from build123d import *

# Parameters (mm, degrees)
SKETCH1_R           = 2.921
SKETCH1_R_2         = 14.0335
SKETCH1_R_3         = 10.8585
SKETCH1_R_4         = 2.4892
SKETCH1_R_5         = 12.3825
BOSS_EXTRUDE1_DEPTH = 6.35
SKETCH2_W           = 6.35
SKETCH2_H           = 6.35
SKETCH2_H_2         = 16.217729686
SKETCH2_R           = 2.15265
CUT_EXTRUDE2_DEPTH  = 196.570791382
FILLET1_R           = 2.54


with BuildPart() as part:
    # Sketch1 → Boss-Extrude1 (new body)
    with BuildSketch(Plane(origin=(0, 0, 0), x_dir=(1, 0, 0), z_dir=(0, 1, 0))):
        with BuildLine():
            ThreePointArc((-168.788743889, 72.590962133), (-181.488743889, 59.890962122), (-168.788743866, 47.190962133))
            Line((-168.788743866, 47.190962133), (-145.58139547, 45.094655563))
            Line((-145.58139547, 45.094655563), (-93.510572414, -45.094655563))
            Line((-93.510572414, -45.094655563), (-105.98261767, -48.892439505))
            ThreePointArc((-105.98261767, -48.892439505), (-111.899875664, -63.177964006), (-99.63261767, -72.590962133))
            Line((-99.63261767, -72.590962133), (47.56445351, -72.590962133))
            Line((47.56445351, -72.590962133), (47.56445351, 72.590962133))
            Line((47.56445351, 72.590962133), (-168.788743889, 72.590962133))
        make_face()
        with Locations(Location((-168.788743889, 59.890962133, 0), (0, 0, 270))):
            Circle(SKETCH1_R, mode=Mode.SUBTRACT)
        with Locations(Location((20.56425351, -34.490962133, 0), (0, 0, 270))):
            Circle(SKETCH1_R_2, mode=Mode.SUBTRACT)
        with Locations(Location((-22.22178223, -28.671379192, 0), (0, 0, 270))):
            Circle(SKETCH1_R_3, mode=Mode.SUBTRACT)
        with Locations(Location((-62.44294649, -9.090962133, 0), (0, 0, 270))):
            Circle(SKETCH1_R_4, mode=Mode.SUBTRACT)
        with Locations(Location((-62.44294649, -34.490962133, 0), (0, 0, 270))):
            Circle(SKETCH1_R_5, mode=Mode.SUBTRACT)
        with Locations(Location((-62.44294649, -59.890962133, 0), (0, 0, 270))):
            Circle(SKETCH1_R_4, mode=Mode.SUBTRACT)
        with Locations(Location((-99.63261767, -59.890962133, 0), (0, 0, 270))):
            Circle(SKETCH1_R, mode=Mode.SUBTRACT)
    extrude(amount=BOSS_EXTRUDE1_DEPTH)

    # Sketch2 → Cut-Extrude2 (cut, through all)
    with BuildSketch(Plane(origin=(0, 6.35, 0), x_dir=(1, 0, 0), z_dir=(0, 1, 0))):
        Polygon((47.56445351, 66.240962133), (41.21445351, 66.240962133), (41.21445351, 50.023232447), (41.21445351, 43.673232447), (41.21445351, -29.703590933), (47.56445351, -39.813704084), align=None)
        with Locations((44.38945351, 69.415962133)):
            Rectangle(SKETCH2_W, SKETCH2_H)
        with Locations((38.03945351, 58.13209729)):
            Rectangle(SKETCH2_W, SKETCH2_H_2)
        with Locations((38.03945351, 69.415962133)):
            Rectangle(SKETCH2_W, SKETCH2_H)
        Polygon((34.86445351, 72.590962133), (-23.035115437, 72.590962133), (-19.04678223, 66.240962133), (34.86445351, 66.240962133), align=None)
        Polygon((34.86445351, 66.240962133), (-19.04678223, 66.240962133), (-8.860686193, 50.023232447), (34.86445351, 50.023232447), align=None)
        Polygon((34.86445351, 50.023232447), (-8.860686193, 50.023232447), (-4.872352987, 43.673232447), (34.86445351, 43.673232447), align=None)
        with Locations((38.03945351, 46.848232447)):
            Rectangle(SKETCH2_W, SKETCH2_H)
        Polygon((34.86445351, 43.673232447), (-4.872352987, 43.673232447), (10.866061277, 18.615413703), (34.86445351, -19.593477782), align=None)
        with BuildLine():
            Line((41.21445351, 43.673232447), (34.86445351, 43.673232447))
            Line((34.86445351, 43.673232447), (34.86445351, -19.593477782))
            ThreePointArc((34.86445351, -19.593477782), (38.05130715, -23.507624068), (40.193418442, -28.077956276))
            Line((40.193418442, -28.077956276), (41.21445351, -29.703590933))
            Line((41.21445351, -29.703590933), (41.21445351, 43.673232447))
        make_face()
        Polygon((47.56445351, -72.590962133), (47.56445351, -39.813704084), (41.21445351, -29.703590933), (41.21445351, -34.490962133), (41.21445351, -66.240962133), (41.21445351, -72.590962133), align=None)
        with Locations(Location((-94.739455539, 46.848232447, 0), (0, 0, 270))):
            Circle(SKETCH2_R)
        with Locations(Location((-22.22178223, 46.848232447, 0), (0, 0, 270))):
            Circle(SKETCH2_R)
        with Locations(Location((2.800077171, 13.549298288, 0), (0, 0, 270))):
            Circle(SKETCH2_R)
        with Locations(Location((1.51425351, -59.890962133, 0), (0, 0, 270))):
            Circle(SKETCH2_R)
        with BuildLine():
            ThreePointArc((40.193418442, -28.077956276), (38.05130715, -23.507624068), (34.86445351, -19.593477782))
            Line((34.86445351, -19.593477782), (40.193418442, -28.077956276))
        make_face()
    extrude(amount=-CUT_EXTRUDE2_DEPTH, mode=Mode.SUBTRACT)

    # Fillet1
    fillet1_edges = [part.edges().sort_by_distance(p)[0] for p in [
        (-93.510572414, 3.175, 45.094655563),
        (-145.58139547, 3.175, -45.094655563),
        (-23.035115437, 3.175, -72.590962133),
        (41.21445351, 3.175, 72.590962133),
        (41.21445351, 3.175, 29.703590933),
    ]]
    fillet(fillet1_edges, radius=FILLET1_R)


solid = part.part
Verification items for the finished model (mm, model axes). A direction names the side the tool comes from. Coordinates: 2 decimals unless noted, no trailing zeros. Order: outer loops, then holes, each group sorted by start corner. A loop starts at its lowest first (then second) coordinate and runs counter-clockwise, first axis right, second up. Notation, with made-up numbers: M 69.25,-19.5 L 73.25,-19.5 A7 ccw 73.25,-6.5 Z; hole C 51.5,-5.5 d10. An arc over 180 degrees is marked long. One line per item, written item: value. Start each with the question number.
Item 1: Sectioned sample at A-A (x = -71.5). Enter the section's corners in (y, z).
Item 2: Scan lines: probe 1 along X at (y, z) = (4.25, 60); probe 2 along X at (y, z) = (3.5, 34); probe 3 along Z at (x, y) = (-26, 2.75). Record each from-to range of solid material in increasing order.
Item 3: Sectioned sample at C-C (x = -152). Enter the section's corners in (y, z).
Item 4: Sectioned sample at B-B (y = 3.75). Count the separate pieces of the cut face and the enclosed holes in it, then the cut area to 3 significant figures.
Item 5: Access from +Z, -Z, +X, -X, +Y, -Y to the whole of each face (thin tool, end or side, straight path). Record for faces 1 (the cylindrical face through (-64.873, 3.131, 8.551)), 2 (the flat face through (-120.364, 3.131, -1.418)).
Item 6: Mould release check, pull along Z, two halves, no side actions. Record for faces 3 (the flat face through (-31, 3, 72.591)), 4 (the cylindrical face through (-28.829, 3.131, 20.054)), 5 (the flat face through (-72, 6.35, -1)): released by +Z, released by -Z, zero draft, split by the parting line, or undercut.
Item 7: Sectioned sample at D-D (z = -6). Enter the section's corners in (x, y), then the cut area to 3 significant figures.
Item 8: Gauge pin test, flat end, axial feed: pin 1 (1 mm diameter, centred on y = 2.5, z = -57.5, fed in from -X). Record the tip position at first contact, or that the pin passes through.
Conclusion:
1. outline: M 0,-72.59 L 6.35,-72.59 L 6.35,26.05 L 0,26.05 Z; M 0,42.93 L 6.35,42.93 L 6.35,72.59 L 0,72.59 Z
2. probe 1: x = -112.33 to -102.55, -96.71 to -64.93, -59.96 to -0.64, 3.66 to 41.21
2. probe 2: x = -99.92 to -74.82, -50.07 to -31.68, -12.76 to 6.54, 34.59 to 41.21
2. probe 3: z = -72.59 to 18.49, 38.85 to 72.59
3. outline: M 0,-72.59 L 6.35,-72.59 L 6.35,-45.67 L 0,-45.67 Z
4. separate pieces: 1
4. enclosed holes: 11
4. area: 19,700 mm^2
5. face 1: +Y, -Y
5. face 2: -X, +Y, -Y
6. face 3: released by +Z
6. face 4: undercut
6. face 5: zero draft
7. outline: M -123.01,0 L 18.79,0 L 18.79,6.35 L -123.01,6.35 Z
7. area: 900 mm^2
8. pin 1: stops at x = -181.35
